Part print with two shaded views. Sizes in mm from the minimum x, y, z corner. A direction names the side the tool comes from. Round coordinates to 2 decimals unless told otherwise and drop trailing zeros. Write each loop counter-clockwise with the first axis right and the second up, starting at its lowest first coordinate (ties: lowest second). Pieces come first, ordered by that corner, then holes. Notation, with made-up numbers: M -31,56 L 21,56 A20 ccw 21,84 Z; hole C 83.5,15.5 d2. An arc over 180 degrees is marked long. Use one line per item in the form item = value. Start each with the question number.
Item 1: Cut at C-C, the plane z = 32. Give the cut face in (x, y), then the cut area to 3 significant figures.
Item 2: Cut at D-D, the plane x = 9.5. Give the cut face in (y, z), then the cut area to 3 significant figures.
Item 3: Cut at B-B, the plane x = 6.5. Give the cut face in (y, z), then the cut area to 3 significant figures.
Item 4: Which spindle directions (+Z, -Z, +X, -X, +Y, -Y) get a long thin tool onto all of the face, cutting with end or side? Do the marked faces 1 and 2. Say none if no direction does.
Item 5: Cut at A-A, the plane y = 5.5. Give the cut face in (x, z).
Item 6: Probe L1, parallel to Y at x = 6.5, z = 30.5; L2, parallel to Z at x = 5.75, y = 7; L3, parallel to Y at x = 6.5, z = 32. List the from-to ranges inside material, lowest first.
Item 7: Flat gauge pins, fed straight in: pin 1 Ø3 at (x, y) = (6.5, 27.5) entering from -Z; pin 2 Ø4 at (x, z) = (6.5, 5.5) entering from -Y; pin 3 Ø1 at (x, z) = (8.5, 18) entering from -Y. Where does each tip first touch, or does it go through?
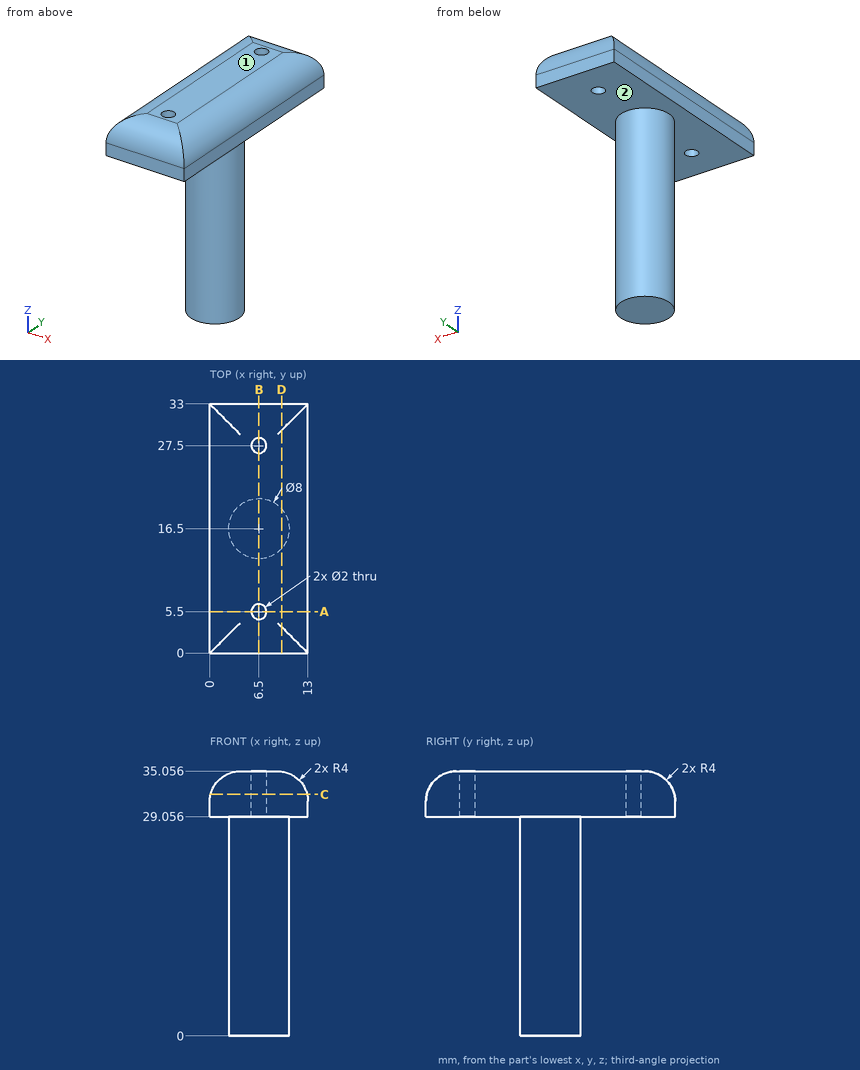
Model answer:
q1.outline = M 0.11,0.11 L 12.89,0.11 L 12.89,32.89 L 0.11,32.89 Z; hole C 6.5,5.5 d2; hole C 6.5,27.5 d2
q1.area = 412 mm²
q2.outline = M 0,29.06 L 13.85,29.06 L 13.85,0 L 19.15,0 L 19.15,29.06 L 33,29.06 L 33,31.06 A4 ccw 29.5,35.02 L 3.5,35.02 A4 ccw 0,31.06 Z
q2.area = 344 mm²
q3.outline = M 0,29.06 L 4.5,29.06 L 4.5,35.06 L 4,35.06 A4 ccw 0,31.06 Z; M 6.5,29.06 L 12.5,29.06 L 12.5,0 L 20.5,0 L 20.5,29.06 L 26.5,29.06 L 26.5,35.06 L 6.5,35.06 Z; M 28.5,29.06 L 33,29.06 L 33,31.06 A4 ccw 29,35.06 L 28.5,35.06 Z
q3.area = 400 mm²
q4.face_1 = +Z, +X, -X, +Y, -Y
q4.face_2 = -Z
q5.outline = M 0,29.06 L 5.5,29.06 L 5.5,35.06 L 4,35.06 A4 ccw 0,31.06 Z; M 7.5,29.06 L 13,29.06 L 13,31.06 A4 ccw 9,35.06 L 7.5,35.06 Z
q6.L1 = 0 to 4.5, 6.5 to 26.5, 28.5 to 33
q6.L2 = 29.06 to 35.06
q6.L3 = 0.11 to 4.5, 6.5 to 26.5, 28.5 to 32.89
q7.pin_1 = 29.06
q7.pin_2 = 12.5
q7.pin_3 = 12.79
